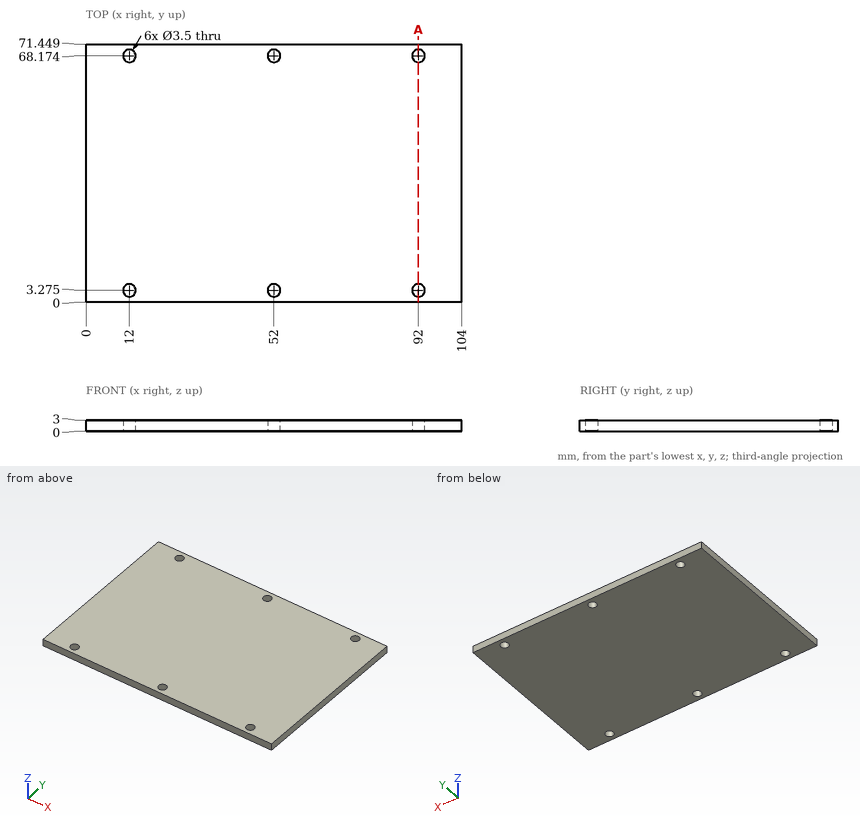
Geometry: see drawing. Coordinates: mm, zero at the bounding-box minimum. Give positions to 0.01 mm unless a question says otherwise; leave off trailing zeros.
1. Cut plane A-A (x = 92). State how many separate pieces and enclosed holes the cut face has, and give its area (3 significant figures).
Computed:
separate pieces: 3
enclosed holes: 0
area: 193 mm2
2. Pin query (flat end, axial travel): pin 1 Ø3 at (x, y) = (92, 3.28) entering from +Z. Return the tip coordinate at first contact, or that it passes through.
Computed:
pin 1: passes through
3. Line query: probe 1 along Y at (x, z) = (53, 1.7). Output: solid intervals per line, ascending.
Computed:
probe 1: y = 0 to 1.84, 4.71 to 66.74, 69.61 to 71.45
